```python
from build123d import *

# Parameters (mm, degrees)
SKETCH1_W           = 144.78
SKETCH1_H           = 144.78
BOSS_EXTRUDE1_DEPTH = 5.08
SKETCH3_W           = 5.08
SKETCH3_H           = 28.956
SKETCH3_W_2         = 28.956
SKETCH3_H_2         = 5.08
CUT_EXTRUDE1_DEPTH  = 205.812849206
CUT_EXTRUDE3_DEPTH  = 205.812849206


with BuildPart() as part:
    # Sketch1 → Boss-Extrude1 (new body)
    with BuildSketch(Plane.XY):
        with Locations((72.39, 72.39)):
            Rectangle(SKETCH1_W, SKETCH1_H)
    extrude(amount=BOSS_EXTRUDE1_DEPTH)

    # Sketch3 → Cut-Extrude1 (cut, through all)
    with BuildSketch(Plane.XY.offset(5.08)):
        with Locations((2.54, 101.346)):
            Rectangle(SKETCH3_W, SKETCH3_H)
        with Locations((2.54, 43.434)):
            Rectangle(SKETCH3_W, SKETCH3_H)
        with Locations((142.24, 101.346)):
            Rectangle(SKETCH3_W, SKETCH3_H)
        with Locations((142.24, 43.434)):
            Rectangle(SKETCH3_W, SKETCH3_H)
        with Locations((43.434, 142.24)):
            Rectangle(SKETCH3_W_2, SKETCH3_H_2)
        with Locations((101.346, 142.24)):
            Rectangle(SKETCH3_W_2, SKETCH3_H_2)
        with Locations((43.434, 2.54)):
            Rectangle(SKETCH3_W_2, SKETCH3_H_2)
        with Locations((101.346, 2.54)):
            Rectangle(SKETCH3_W_2, SKETCH3_H_2)
    extrude(amount=-CUT_EXTRUDE1_DEPTH, mode=Mode.SUBTRACT)

    # Sketch7 → Cut-Extrude3 (cut, through all)
    with BuildSketch(Plane.XY.offset(5.08)):
        Polygon((72.39, 129.54), (94.26035816, 125.189715283), (93.288342241, 122.84306127), (72.39, 127), align=None)
        Polygon((129.54, 72.39), (125.189715283, 50.51964184), (122.84306127, 51.491657759), (127, 72.39), align=None)
        Polygon((72.39, 15.24), (50.51964184, 19.590284717), (51.491657759, 21.93693873), (72.39, 17.78), align=None)
        Polygon((17.78, 72.39), (21.93693873, 93.288342241), (19.590284717, 94.26035816), (15.24, 72.39), align=None)
    extrude(amount=-CUT_EXTRUDE3_DEPTH, mode=Mode.SUBTRACT)


solid = part.part
```
Geometry: final body of the model. Coordinates: model frame, mm. A direction names the side the tool comes from. Give positions to 0.01 mm unless a question says otherwise; leave off trailing zeros. Loops run counter-clockwise (first coordinate to the right, second up) from the corner with the lowest first, then second, coordinate; pieces in that order, holes last. Notation, with made-up numbers: (-4, 31) -> (9, 31) arc R27 ccw to (9, 66) -> close; hole circle Ø2 at (57, 55). An arc over 180 degrees is marked (long way). Return JSON: item names as keys, results as strings.
Item 1: Mould query, pull axis X, two halves, no side actions, for faces 4 (the flat face through (61.79, 19.89, 2.58)), 5 (the flat face through (144.78, 14, 3)), 6 (the flat face through (3, 115.824, 3)), 7 (the flat face through (57.912, 3, 3)). Classes: released by +X, released by -X, zero draft, split by the parting line, or undercut.
Filled in:
{"face 4": "undercut", "face 5": "released by +X", "face 6": "zero draft", "face 7": "undercut"}
Item 2: Pin query (flat end, axial travel): P1, Ø1.5, axis at y = 98.5, z = 3.5, coming from the -X side; P2, Ø3, axis at x = 128.5, z = 2.5, coming from the -Y side; P3, Ø1.5, axis at y = 41, z = 1.5, coming from the +X side. Return the tip coordinate at first contact, or that it passes through.
Filled in:
{"P1": "x = 5.08", "P2": "y = 0", "P3": "x = 139.7"}
Item 3: Section A-A, the plane x = 84. Output: boundary loops of the cut face in (y, z).
Filled in:
{"outline": "(0, 0) -> (124.69, 0) -> (124.69, 5.08) -> (0, 5.08) -> close; (127.23, 0) -> (144.78, 0) -> (144.78, 5.08) -> (127.23, 5.08) -> close"}
Item 4: Line query: line 1 (X direction, y = 109, z = 4.7); line 2 (X direction, y = 82, z = 0.4); line 3 (Y direction, x = 67.5, z = 0.65). Output: solid intervals per line, ascending.
Filled in:
{"line 1": "5.08 to 139.7", "line 2": "0 to 17.15, 19.69 to 144.78", "line 3": "0 to 16.21, 18.75 to 144.78"}
Item 5: Access query for faces 1 (the flat face through (86.868, 142, 3)), 2 (the flat face through (142, 115.824, 3)), 3 (the flat face through (127.395, 61.608, 2.576)). Directions: +Z, -Z, +X, -X, +Y, -Y. A direction counts if a zero-diameter tool reaches every point of the face in a straight line with its end or side. Return the directions, or none.
Filled in:
{"face 1": "+Z, -Z, +Y", "face 2": "+Z, -Z, +X", "face 3": "+Z, -Z"}
Item 6: Section B-B, the plane y = 105.5. Output: boundary loops of the cut face in (x, z), plus the area to 3 significant figures.
Filled in:
{"outline": "(5.08, 0) -> (139.7, 0) -> (139.7, 5.08) -> (5.08, 5.08) -> close", "area": "684 mm^2"}
Item 7: Section C-C, the plane z = 3.9. Count the separate pieces of the cut face and the enclosed holes in it, plus the area to 3 significant figures.
Filled in:
{"separate pieces": "1", "enclosed holes": "4", "area": "19,600 mm^2"}
